```python
from build123d import *

# Parameters (mm, degrees)
F1_DEPTH = 0.5
F2_DEPTH = 25
F3_R     = 2.9
F4_DEPTH = 0.501
F6_DEPTH = 0.5


# Not quite as in the source:
# - a feature names something its author has since deleted; it is built from what else it names


with BuildPart() as f1:
    # F0 (on Top) → F1 (new body)
    with BuildSketch(Plane.XY):
        with BuildLine():
            Line((4.0961373656, 12.3378141776), (-4.8678095704, 15.3138321001))
            Line((-4.8678095704, 15.3138321001), (-10.4681826882, 7.7082521499))
            ThreePointArc((-10.4681826882, 7.7082521499), (-3.9381406197, 12.3891504333), (4.0961373656, 12.3378141776))
        make_face()
    extrude(amount=F1_DEPTH)



with BuildPart() as f1b:
    # F0 (on Top) → F1, piece 2 (new body)
    with BuildSketch(Plane.XY):
        with BuildLine():
            Line((13.0600839256, 9.36179638), (4.0961373656, 12.3378141776))
            ThreePointArc((4.0961373656, 12.3378141776), (9.7852826172, 8.5585188031), (12.7733744664, 2.41679638))
            Line((12.7733744664, 2.41679638), (13.01569776, 2.4152179267))
            Line((13.01569776, 2.4152179267), (13.0600839256, 9.36179638))
        make_face()
        with BuildLine():
            Line((13.01569776, 2.4152179267), (12.7733744664, 2.41679638))
            ThreePointArc((12.7733744664, 2.41679638), (12.9432196161, 1.2136992909), (13, 0))
            ThreePointArc((13, 0), (12.9999336569, -0.0415321088), (12.9997346283, -0.0830637936))
            Line((12.9997346283, -0.0830637936), (13.01569776, 2.4152179267))
        make_face()
        with BuildLine():
            Line((21.6332001204, 2.3590849609), (13.01569776, 2.4152179267))
            Line((13.01569776, 2.4152179267), (12.9997346283, -0.0830637936))
            Line((12.9997346283, -0.0830637936), (12.9837495259, -2.5847840032))
            Line((12.9837495259, -2.5847840032), (21.6006561013, -2.640828477))
            ThreePointArc((21.6006561013, -2.640828477), (21.374282177, -0.1392923959), (21.6332001204, 2.3590849609))
        make_face()
        with BuildLine():
            ThreePointArc((12.7407636764, -2.58320362), (9.6739656437, -8.6841458259), (3.9381407553, -12.3891503902))
            Line((3.9381407553, -12.3891503902), (12.9393853324, -9.5279237416))
            Line((12.9393853324, -9.5279237416), (12.9837495259, -2.5847840032))
            Line((12.9837495259, -2.5847840032), (12.7407636764, -2.58320362))
        make_face()
        with BuildLine():
            Line((12.9837495259, -2.5847840032), (12.9997346283, -0.0830637936))
            ThreePointArc((12.9997346283, -0.0830637936), (12.9308154434, -1.3394073199), (12.7407636764, -2.58320362))
            Line((12.7407636764, -2.58320362), (12.9837495259, -2.5847840032))
        make_face()
        with BuildLine():
            ThreePointArc((47.3740068068, -0.2239065181), (35.6719885241, 12.7111328503), (21.6332001204, 2.3590849609))
            Line((21.6332001204, 2.3590849609), (30.0602249194, 2.304192734))
            ThreePointArc((30.0602249194, 2.304192734), (35.6837950651, 4.6014903276), (39.3740068068, -0.2239065181))
            ThreePointArc((39.3740068068, -0.2239065181), (35.6523599398, -5.0577262569), (30.0276814999, -2.6956379611))
            Line((30.0276814999, -2.6956379611), (21.6006561013, -2.640828477))
            ThreePointArc((21.6006561013, -2.640828477), (35.5877697221, -13.1671201679), (47.3740068068, -0.2239065181))
        make_face()
        with BuildLine():
            Line((30.0602249194, 2.304192734), (21.6332001204, 2.3590849609))
            ThreePointArc((21.6332001204, 2.3590849609), (21.374282177, -0.1392923959), (21.6006561013, -2.640828477))
            Line((21.6006561013, -2.640828477), (30.0276814999, -2.6956379611))
            ThreePointArc((30.0276814999, -2.6956379611), (29.374112718, -0.1913626859), (30.0602249194, 2.304192734))
        make_face()
        with BuildLine():
            Line((32.7319335315, 2.286789672), (30.0602249194, 2.304192734))
            ThreePointArc((30.0602249194, 2.304192734), (29.374112718, -0.1913626859), (30.0276814999, -2.6956379611))
            Line((30.0276814999, -2.6956379611), (32.6993904313, -2.7130147911))
            ThreePointArc((32.6993904313, -2.7130147911), (31.3740703529, -0.2043803079), (32.7319335315, 2.286789672))
        make_face()
        with BuildLine():
            ThreePointArc((37.3740068068, -0.2239065181), (35.80120339, 2.4148640125), (32.7319335315, 2.286789672))
            Line((32.7319335315, 2.286789672), (34.3740068068, 2.2760934819))
            Line((34.3740068068, 2.2760934819), (34.3740068068, -2.7239065181))
            Line((34.3740068068, -2.7239065181), (32.6993904313, -2.7130147911))
            ThreePointArc((32.6993904313, -2.7130147911), (35.7839980964, -2.8719104009), (37.3740068068, -0.2239065181))
        make_face()
        with BuildLine():
            Line((34.3740068068, 2.2760934819), (32.7319335315, 2.286789672))
            ThreePointArc((32.7319335315, 2.286789672), (31.3740703529, -0.2043803079), (32.6993904313, -2.7130147911))
            Line((32.6993904313, -2.7130147911), (34.3740068068, -2.7239065181))
            Line((34.3740068068, -2.7239065181), (34.3740068068, 2.2760934819))
        make_face()
    extrude(amount=F1_DEPTH)

    # F0 (on Top) → F2 (join)
    with BuildSketch(Plane.XY):
        with BuildLine():
            ThreePointArc((39.3740068068, -0.2239065181), (35.6837950651, 4.6014903276), (30.0602249194, 2.304192734))
            Line((30.0602249194, 2.304192734), (32.7319335315, 2.286789672))
            ThreePointArc((32.7319335315, 2.286789672), (35.80120339, 2.4148640125), (37.3740068068, -0.2239065181))
            ThreePointArc((37.3740068068, -0.2239065181), (35.7839980964, -2.8719104009), (32.6993904313, -2.7130147911))
            Line((32.6993904313, -2.7130147911), (30.0276814999, -2.6956379611))
            ThreePointArc((30.0276814999, -2.6956379611), (35.6523599398, -5.0577262569), (39.3740068068, -0.2239065181))
        make_face()
        with BuildLine():
            Line((32.7319335315, 2.286789672), (30.0602249194, 2.304192734))
            ThreePointArc((30.0602249194, 2.304192734), (29.374112718, -0.1913626859), (30.0276814999, -2.6956379611))
            Line((30.0276814999, -2.6956379611), (32.6993904313, -2.7130147911))
            ThreePointArc((32.6993904313, -2.7130147911), (31.3740703529, -0.2043803079), (32.7319335315, 2.286789672))
        make_face()
    extrude(amount=F2_DEPTH)

    # F3 (on face) → F4 (cut, through all)
    with BuildSketch(Plane.XY.offset(0.5)):
        with Locations((34.3740068068, -0.2239065181)):
            Circle(F3_R)
    extrude(amount=-F4_DEPTH, mode=Mode.SUBTRACT)


with BuildPart() as f1c:
    # F0 (on Top) → F1, piece 3 (new body)
    with BuildSketch(Plane.XY):
        with BuildLine():
            ThreePointArc((3.9381407553, -12.3891503902), (-4.096137147, -12.3378142502), (-10.5658298597, -7.5738523471))
            Line((-10.5658298597, -7.5738523471), (-5.0631039967, -15.2503770945))
            Line((-5.0631039967, -15.2503770945), (3.9381407553, -12.3891503902))
        make_face()
    extrude(amount=F1_DEPTH)


with BuildPart() as f1_1:
    add(f1.part)

    add(f1b.part)  # F6 merges F1b

    add(f1c.part)  # F6 merges F1c
    # F5 (on face) → F6 (join, through all)
    with BuildSketch(Plane.XY):
        Polygon((-4.8678095704, 15.3138321001), (4.0961371776, 12.3378142401), (13.0600839256, 9.36179638), (13.0735205907, 11.4646779011), (-3.6208963346, 17.0072011144), align=None)
        Polygon((-5.0631039967, -15.2503770945), (-3.8421437919, -16.9585881221), (12.9230595755, -11.6340152664), (12.9393853324, -9.5279237416), (3.9381406679, -12.389150418), align=None)
    extrude(amount=F6_DEPTH)


solid = f1_1.part
```
Geometry check sheet. Reference: the model listing, model coordinates, mm. Coordinates: 2 decimals unless noted, no trailing zeros. Order: outer loops, then holes, each group sorted by start corner. A loop starts at its lowest first (then second) coordinate and runs counter-clockwise, first axis right, second up. Notation, with made-up numbers: (55.25, -15) - (87.25, -15) arc R14 ccw to (87.25, 4) - close; hole circle Ø9 at (63.25, 5). An arc over 180 degrees is marked (long way). Answer in a Markdown table with one row per item. Add a question column.
1. Section check B-B (x = -2). Enter the section's corners in (y, z).
2. Material ranges on L1, parallel to Z at x = 5, y = 14; L2, parallel to Y at x = 35, z = 5.75; L3, parallel to X at y = 3.5, z = 10, recorded low to high. Write a range as [from, to].
3. Section check A-A (y = -1). Enter the section's corners in (x, z), plus the area to 3 significant figures.
4. Section check D-D (y = -6). Enter the section's corners in (x, z), plus the area to 3 significant figures.
5. Gauge pin test, flat ends, axial feed: pin 1 Ø4.5 at (x, y) = (34.37, -0.22) entering from -Z; pin 2 Ø12 at (x, z) = (31.5, 13) entering from -Y; pin 3 Ø12 at (y, z) = (0, 19) entering from -X; pin 4 Ø6 at (y, z) = (-0.5, 12.5) entering from +X. Record the tip position at first contact, or that the pin passes through.
6. Draft check along X on faces 1 (the face through (4.84, 14.2, 0.25)), 2 (the face through (37, -2, 25)), 3 (the face through (4.423, -14.334, 0.246)). Enter one of: +X half, -X half, draft (parallel to the pull), parting line (faces both ways), or undercut.
7. Section check C-C (z = 7.75). Enter the section's corners in (x, y).
Data:
| question | item | result |
|---|---|---|
| 1 | outline | (-16.37, 0) - (-12.85, 0) - (-12.85, 0.5) - (-16.37, 0.5) - close; (12.85, 0) - (16.47, 0) - (16.47, 0.5) - (12.85, 0.5) - close |
| 2 | L1 | z = [0, 0.5] |
| 2 | L2 | y = [-5.18, -3.16], [2.71, 4.74] |
| 2 | L3 | x = [31.04, 37.71] |
| 3 | outline | (12.96, 0) - (31.58, 0) - (31.58, 0.5) - (31.48, 0.5) - (31.48, 25) - (29.43, 25) - (29.43, 0.5) - (12.96, 0.5) - close; (37.17, 0) - (47.35, 0) - (47.35, 0.5) - (39.31, 0.5) - (39.31, 25) - (37.27, 25) - (37.27, 0.5) - (37.17, 0.5) - close |
| 3 | area | 114 mm² |
| 4 | outline | (11.53, 0) - (12.96, 0) - (12.96, 0.5) - (11.53, 0.5) - close; (22.73, 0) - (46.02, 0) - (46.02, 0.5) - (22.73, 0.5) - close |
| 4 | area | 12.4 mm² |
| 5 | pin 1 | passes through |
| 5 | pin 2 | stops at y = -5.22 |
| 5 | pin 3 | stops at x = 29.37 |
| 5 | pin 4 | stops at x = 39.37 |
| 6 | face 1 | undercut |
| 6 | face 2 | draft |
| 6 | face 3 | undercut |
| 7 | outline | circle Ø10 at (34.37, -0.22); hole circle Ø6 at (34.37, -0.22) |
